```python
from build123d import *

# Parameters (mm, degrees)
SALIENTE_EXTRUIR1_DEPTH = 50
CORTAR_EXTRUIR1_DEPTH   = 30
SALIENTE_EXTRUIR2_REACH = 69.091
CROQUIS4_R              = 12.5
CROQUIS4_R_2            = 6
SALIENTE_EXTRUIR3_DEPTH = 15
CROQUIS5_R              = 6
CORTAR_EXTRUIR2_DEPTH   = 68.09125606
CORTAR_EXTRUIR3_DEPTH   = 101
SALIENTE_EXTRUIR5_REACH = 82.311
CORTAR_EXTRUIR4_DEPTH   = 5
CROQUIS9_R              = 7.5
CORTAR_EXTRUIR5_DEPTH   = 76.310889132


with BuildPart() as part:
    # Croquis1 → Saliente-Extruir1 (new body, symmetric)
    with BuildSketch(Plane.XY):
        Polygon((0, 0), (0, 25), (100, 25), (100, 40), (200, 40), (200, 0), (150, 0), (150, -10), (112.5, -10), (112.5, 0), (87.5, 0), (87.5, -10), (50, -10), (50, 0), align=None)
    extrude(amount=SALIENTE_EXTRUIR1_DEPTH, both=True)

    # Croquis2 → Cortar-Extruir1 (cut)
    with BuildSketch(Plane.XY.offset(50)):
        with BuildLine():
            Line((78.205505282, 25), (100, 25))
            Line((100, 25), (100, 40))
            Line((100, 40), (140, 40))
            ThreePointArc((140, 40), (111.794494718, 21.411010565), (78.205505282, 25))
        make_face()
    extrude(amount=-CORTAR_EXTRUIR1_DEPTH, mode=Mode.SUBTRACT)

    # Saliente-Extruir2: up to this face of the body (flat: up to its plane)
    saliente_extruir2_end = Plane(part.part.faces().sort_by_distance((47.264467122, 25, -2.448514344))[0])
    # Croquis3 → Saliente-Extruir2 (add, up to the picked face)
    with BuildSketch(Plane(origin=(0, 38.145245781, 13.883734043), x_dir=(-1, 0, 0), z_dir=(0, 0.939692621, 0.342020143)), mode=Mode.PRIVATE) as saliente_extruir2_sk1:
        with BuildLine():
            Line((-15, 38.434127456), (-15, -1.565872544))
            ThreePointArc((-15, -1.565872544), (-40, -26.565872544), (-65, -1.565872544))
            Line((-65, -1.565872544), (-65, 38.434127456))
            Line((-65, 38.434127456), (-15, 38.434127456))
        make_face()
    saliente_extruir2_tool1 = split(extrude(saliente_extruir2_sk1.sketch, amount=-SALIENTE_EXTRUIR2_REACH, mode=Mode.PRIVATE), bisect_by=saliente_extruir2_end, keep=Keep.BOTH, mode=Mode.PRIVATE)
    add(saliente_extruir2_tool1.solids().sort_by(Axis((40, 35.287462, 21.735431), (0, -0.939692621, -0.342020143)))[0])

    # Croquis4 → Saliente-Extruir3 (add)
    with BuildSketch(Plane(origin=(0, 38.145245781, 13.883734043), x_dir=(1, 0, 0), z_dir=(0, 0.939692621, 0.342020143))):
        with Locations(Location((40, 1.565872544, 0), (0, 0, 270))):  # turned: the seam where the file's is
            Circle(CROQUIS4_R)
        with Locations(Location((40, 1.565872544, 0), (0, 0, 270))):  # turned: the seam where the file's is
            Circle(CROQUIS4_R_2, mode=Mode.SUBTRACT)
    extrude(amount=SALIENTE_EXTRUIR3_DEPTH)

    # Croquis5 → Cortar-Extruir2 (cut, through all)
    with BuildSketch(Plane(origin=(0, 38.145245781, 13.883734043), x_dir=(-1, 0, 0), z_dir=(0, 0.939692621, 0.342020143))):
        with Locations(Location((-40, -1.565872544, 0), (0, 0, 90))):  # turned: the seam where the file's is
            Circle(CROQUIS5_R)
    extrude(amount=-CORTAR_EXTRUIR2_DEPTH, mode=Mode.SUBTRACT)

    # Croquis6 → Cortar-Extruir3 (cut, through all)
    with BuildSketch(Plane.XY.offset(50)):
        Polygon((100, 25), (100, 40), (125.980762114, 40), align=None)
    extrude(amount=-CORTAR_EXTRUIR3_DEPTH, mode=Mode.SUBTRACT)

    # Saliente-Extruir5: up to this face of the body (flat: up to its plane)
    saliente_extruir5_end = Plane(part.part.faces().sort_by_distance((164.797670499, 40, -2.108504349))[0])
    # Croquis7 → Saliente-Extruir5 (add, up to the picked face)
    with BuildSketch(Plane(origin=(14.174682453, -24.551270189, 0), x_dir=(0.866025404, 0.5, 0), z_dir=(-0.5, 0.866025404, 0)), mode=Mode.PRIVATE) as saliente_extruir5_sk1:
        with BuildLine():
            Line((99.102540378, 50), (149.102540378, 50))
            ThreePointArc((149.102540378, 50), (184.102540378, 15), (149.102540378, -20))
            Line((149.102540378, -20), (99.102540378, -20))
            Line((99.102540378, -20), (99.102540378, 50))
        make_face()
    saliente_extruir5_tool1 = split(extrude(saliente_extruir5_sk1.sketch, amount=-SALIENTE_EXTRUIR5_REACH, mode=Mode.PRIVATE), bisect_by=saliente_extruir5_end, keep=Keep.BOTH, mode=Mode.PRIVATE)
    add(saliente_extruir5_tool1.solids().sort_by(Axis((133.894705, 44.569117, -15), (0.5, -0.866025404, 0)))[0])

    # Croquis8 → Cortar-Extruir4 (cut)
    with BuildSketch(Plane(origin=(14.174682453, -24.551270189, 0), x_dir=(0.866025404, 0.5, 0), z_dir=(-0.5, 0.866025404, 0))):
        with BuildLine():
            Line((154.102540378, 3.543560763), (154.102540378, -26.456439237))
            Line((154.102540378, -26.456439237), (144.102540378, -26.456439237))
            Line((144.102540378, -26.456439237), (144.102540378, 3.543560763))
            ThreePointArc((144.102540378, 3.543560763), (140.263705614, 6.161165235), (137.646101141, 10))
            Line((137.646101141, 10), (107.646101141, 10))
            Line((107.646101141, 10), (107.646101141, 20))
            Line((107.646101141, 20), (137.646101141, 20))
            ThreePointArc((137.646101141, 20), (140.263705614, 23.838834765), (144.102540378, 26.456439237))
            Line((144.102540378, 26.456439237), (144.102540378, 56.456439237))
            Line((144.102540378, 56.456439237), (154.102540378, 56.456439237))
            Line((154.102540378, 56.456439237), (154.102540378, 26.456439237))
            ThreePointArc((154.102540378, 26.456439237), (157.941375143, 23.838834765), (160.558979616, 20))
            Line((160.558979616, 20), (190.558979616, 20))
            Line((190.558979616, 20), (190.558979616, 10))
            Line((190.558979616, 10), (160.558979616, 10))
            ThreePointArc((160.558979616, 10), (157.941375143, 6.161165235), (154.102540378, 3.543560763))
        make_face()
    extrude(amount=-CORTAR_EXTRUIR4_DEPTH, mode=Mode.SUBTRACT)

    # Croquis9 → Cortar-Extruir5 (cut, through all)
    with BuildSketch(Plane(origin=(16.674682453, -28.881397208, 0), x_dir=(0.866025404, 0.5, 0), z_dir=(-0.5, 0.866025404, 0))):
        with Locations(Location((149.102540378, 15, 0), (0, 0, 180))):  # turned: the seam where the file's is
            Circle(CROQUIS9_R)
    extrude(amount=-CORTAR_EXTRUIR5_DEPTH, mode=Mode.SUBTRACT)


solid = part.part
```
The listing builds one solid part. Answer for the finished solid, in the listing's coordinates (mm). A direction names the side the tool comes from. Coordinates: 2 decimals unless noted, no trailing zeros. Loops run counter-clockwise (first coordinate to the right, second up) from the corner with the lowest first, then second, coordinate; pieces in that order, holes last. Notation, with made-up numbers: (30.5, 9.5) -> (42.5, 9.5) arc R23 ccw to (42.5, 23.5) -> close; hole circle Ø5 at (39, 23.25). An arc over 180 degrees is marked (long way). Use one line per item in the form item = value. Start each with the question number.
Item 1: The part is cut by section A-A on y = -2.5. Determine the outline of the cut face in (x, z).
Item 2: Flat-ended cylindrical pins translate along their axes: pin 1 Ø18 at (x, z) = (162.5, -8.5) entering from +Y; pin 2 Ø4 at (y, z) = (34.5, 34.5) entering from -X; pin 3 Ø5 at (x, y) = (167.5, 57) entering from +Z. Find the tip coordinate at first contact, or state that the pin passes through.
Item 3: The part is cut by section D-D on x = 71. Determine the outline of the cut face in (y, z), then the cut area to 3 significant figures.
Item 4: Consider L1, parallel to X at y = -6, z = -8.5; L2, parallel to Y at x = 98.5, z = 26; L3, parallel to Z at x = 37.5, y = 8. Determine where each line is inside the solid, lowest interval first. Write a range as [from, to].
Item 5: The part is cut by section C-C on y = 27. Count the separate pieces of the cut face and the enclosed holes in it, then the cut area to 3 significant figures.
Item 6: A tool of negligible diameter and unlimited length cuts with its end or side. For faces 1 (the face through (122, 35, -10)), 2 (the face through (45.731, 51.886, 19.988)), 3 (the face through (148.86, 50.37, 7.89)), from which of +Z, -Z, +X, -X, +Y, -Y can it reach the whole face along a straight path? Write none if from no direction.
Item 7: The part is cut by section B-B on z = -39. Determine the outline of the cut face in (x, y), then the cut area to 3 significant figures.
Item 8: The mould has two halves that part along Y. Classify faces 4 (the face through (140.2, 45.37, 8.39)), 5 (the face through (148.86, 50.37, -38.21)), 6 (the face through (121, 35, -20)): released by +Y, released by -Y, zero draft, split by the parting line, or undercut.
Answer key:
q1.outline = (50, -50) -> (87.5, -50) -> (87.5, 50) -> (50, 50) -> close; (112.5, -50) -> (150, -50) -> (150, 50) -> (112.5, 50) -> close
q2.pin_1 = 66.28
q2.pin_2 = 133.07
q2.pin_3 = 12.26
q3.outline = (-10, -50) -> (25, -50) -> (25, 50) -> (-10, 50) -> close
q3.area = 3,500 mm2
q4.L1 = [50, 87.5], [112.5, 150]
q4.L2 = [0, 20.02]
q4.L3 = [-50, -4.56], [7.05, 50]
q5.separate_pieces = 2
q5.enclosed_holes = 3
q5.area = 11,500 mm2
q6.face_1 = +Y
q6.face_2 = +Z, -X, +Y
q6.face_3 = +Z, -Z
q7.outline = (0, 0) -> (50, 0) -> (50, -10) -> (87.5, -10) -> (87.5, 0) -> (112.5, 0) -> (112.5, -10) -> (150, -10) -> (150, 0) -> (200, 0) -> (200, 40) -> (178.49, 40) -> (165.36, 62.74) -> (147.63, 52.5) -> (150.13, 48.17) -> (141.47, 43.17) -> (138.97, 47.5) -> (100, 25) -> (0, 25) -> close
q7.area = 7,600 mm2
q8.face_4 = released by +Y
q8.face_5 = undercut
q8.face_6 = zero draft
